Autodesk Inventor part; units mm, degrees
ref_plane "YZ Plane" through (0, 0, 0) normal (1, 0, 0) x (0, 1, 0)
ref_plane "XZ Plane" through (0, 0, 0) normal (0, 1, 0) x (-1, 0, 0)
ref_plane "XY Plane" through (0, 0, 0) normal (0, 0, 1) x (1, 0, 0)
sketch "Sketch1" plane through (0, 0, 0) normal (0, 0, 1) x (1, 0, 0)
  line L0 (-26.9068, 18.7438) -> (-8.9068, 18.7438)
  line L1 (-8.9068, 18.7438) -> (-8.9068, 0.7438)
  line L2 (-8.9068, 0.7438) -> (-26.9068, 0.7438)
  line L3 (-26.9068, 0.7438) -> (-26.9068, 18.7438)
  point P0 (0, 0)
  dimension "d5" = 18
  dimension "d6" = 18
extrude "Extrusion1" add sketch "Sketch1" along normal blind 9
sketch "Sketch2" plane through (0, 0, 0) normal (0, 0, -1) x (-1, 0, 0)
  line L0 (8.9068, 18.7438) -> (26.9068, 18.7438)
  arc A0 (26.9068, 10.7438) -> (18.9068, 18.7438) centre (18.9068, 10.7438) ccw
  arc A1 (25.9068, 10.7438) -> (18.9068, 17.7438) centre (18.9068, 10.7438) ccw
  line L1 (9.9068, 17.7438) -> (25.9068, 17.7438)
  arc A2 (16.9068, 17.7438) -> (9.9068, 10.7438) centre (16.9068, 10.7438) ccw
  arc A3 (16.9068, 18.7438) -> (8.9068, 10.7438) centre (16.9068, 10.7438) ccw
  line L2 (8.9068, 0.7438) -> (8.9068, 18.7438)
  line L3 (9.9068, 1.7438) -> (9.9068, 17.7438)
  arc A4 (8.9068, 8.7438) -> (16.9068, 0.7438) centre (16.9068, 8.7438) ccw
  arc A5 (9.9068, 8.7438) -> (16.9068, 1.7438) centre (16.9068, 8.7438) ccw
  line L4 (26.9068, 0.7438) -> (8.9068, 0.7438)
  line L5 (25.9068, 1.7438) -> (9.9068, 1.7438)
  arc A6 (18.9068, 0.7438) -> (26.9068, 8.7438) centre (18.9068, 8.7438) ccw
  arc A7 (18.9068, 1.7438) -> (25.9068, 8.7438) centre (18.9068, 8.7438) ccw
  line L6 (25.9068, 17.7438) -> (25.9068, 1.7438)
  line L7 (26.9068, 18.7438) -> (26.9068, 0.7438)
  line L8 (26.6568, 10.4938) -> (26.1568, 10.4938)
  line L9 (26.1568, 10.4938) -> (26.1568, 8.9938)
  line L10 (26.1568, 8.9938) -> (26.6568, 8.9938)
  line L11 (26.6568, 8.9938) -> (26.6568, 10.4938)
  circle A8 centre (17.9068, 9.7438) radius 8.75
  line L12 (17.1568, 17.9938) -> (18.6568, 17.9938)
  line L13 (18.6568, 17.9938) -> (18.6568, 18.4938)
  line L14 (18.6568, 18.4938) -> (17.1568, 18.4938)
  line L15 (17.1568, 18.4938) -> (17.1568, 17.9938)
  line L16 (9.6568, 8.9938) -> (9.6568, 10.4938)
  line L17 (9.6568, 10.4938) -> (9.1568, 10.4938)
  line L18 (9.1568, 10.4938) -> (9.1568, 8.9938)
  line L19 (9.1568, 8.9938) -> (9.6568, 8.9938)
  line L20 (18.6568, 1.4938) -> (17.1568, 1.4938)
  line L21 (17.1568, 1.4938) -> (17.1568, 0.9938)
  line L22 (17.1568, 0.9938) -> (18.6568, 0.9938)
  line L23 (18.6568, 0.9938) -> (18.6568, 1.4938)
  point P0 (0, 0)
  point P1 (18.6568, 18.4616)
  point P2 (17.1568, 18.4616)
  point P3 (9.189, 10.4938)
  point P4 (9.189, 8.9938)
  point P5 (17.1568, 1.026)
  point P6 (18.6568, 1.026)
  point P7 (26.6245, 8.9938)
  point P8 (26.6245, 10.4938)
  dimension "d12" = 1.5
  dimension "d13" = 0.5
  dimension "d14" = 0.25
  dimension "d16" = 0.25
  dimension "d18" = 8
  dimension "d19" = 17.5
  dimension "d22" = 360
fillet "Fillet3" radius 8 8 edges at (-8.9068, 18.7438, 4.5) (-17.9068, 18.7438, 9) (-26.9068, 18.7438, 4.5) (-26.9068, 9.7438, 9) (-8.9068, 9.7438, 9) (-8.9068, 0.7438, 4.5) (-17.9068, 0.7438, 9) (-26.9068, 0.7438, 4.5)
shell "Shell2" thickness 1 removed faces 1 at (-17.5734, 12.7438, 0)
extrude "Extrusion4" cut sketch "Sketch2" against normal blind 2 contours A8 L13 L12 L15 | L17 L16 L19 A8 | A8 L10 L9 L8 | L21 L20 L23 A8
properties part number "McCrea_horny_kos_walle_MIR2" material "Silver"
Can you work these out from the model? Positions are in its coordinate system, mm. A direction names the side the tool comes from. Coordinates: 2 decimals unless noted, no trailing zeros. Write each loop counter-clockwise with the first axis right and the second up, starting at its lowest first coordinate (ties: lowest second). Pieces come first, ordered by that corner, then holes. Notation, with made-up numbers: (-28, -38.5) -> (26, -38.5) arc R10 ccw to (26, -19.5) -> close; hole circle Ø5 at (69, -10). An arc over 180 degrees is marked (long way). Answer as CSV lines item,"result".
1) Will these pins go through, and if not, where does the flat tip stop? P1, Ø2, axis at x = -18.5, z = 6, coming from the -Y side; P2, Ø1.6, axis at x = -18, y = 9.5, coming from the -Z side; P3, Ø1.5, axis at x = -19.5, z = 6.5, coming from the +Y side.
Check result:
P1,"y = 1.82"
P2,"z = 8"
P3,"y = 17.16"
2) On a 3-axis mill with a long thin cutter (end or side, diameter ignored), from which of +Z, -Z, +X, -X, +Y, -Y can I reach the whole of each face in a straight line? I mean faces 5 (the cylindrical face through (-17.893, 15.748, 5.895)), 6 (the cylindrical face through (-11.31, 3.03, 0.51)). Say none if no direction works.
Check result:
face 5,"-Z"
face 6,"+Z, -Z, +X, -Y"
3) If we section it at C-C on x = -11.25: Please give me the cut outline in (y, z), then the cut area to 3 significant figures.
Check result:
outline,"(3.09, 0) -> (4.62, 0) -> (4.62, 1) arc R4.12 cw to (8.74, 5.12) -> (10.74, 5.12) arc R4.12 cw to (14.87, 1) -> (14.87, 0) -> (16.4, 0) -> (16.4, 1) arc R5.66 ccw to (10.74, 6.66) -> (8.74, 6.66) arc R5.66 ccw to (3.09, 1) -> close"
area,"29.7 mm²"
4) If we section it at D-D on z = 8.5: Please give me the cut outline in (x, y), then the cut area to 3 significant figures.
Check result:
outline,"(-21.69, 8.74) arc R2.78 ccw to (-18.91, 5.96) -> (-16.91, 5.96) arc R2.78 ccw to (-14.12, 8.74) -> (-14.12, 10.74) arc R2.78 ccw to (-16.91, 13.53) -> (-18.91, 13.53) arc R2.78 ccw to (-21.69, 10.74) -> close"
area,"50.6 mm²"
5) If I drill on line 1 (X direction, y = 10.75, z = 6.25); line 2 (X direction, y = 14.25, z = 5.5); line 3 (Y direction, x = -17.75, z = 3.5), over which ranges is the centre line in solid material (lowest first)? Write a range as from..to.
Check result:
line 1,"-24.94..-23.54, -12.28..-10.87"
line 2,"-24.52..-22.96, -12.85..-11.3"
line 3,"1.14..2.21, 17.28..18.34"
6) If we mould it in two halves opening along X, with no side actions, what happens to faces 1 (the flat face through (-26.157, 10, 1)), 2 (the cylindrical face through (-11.19, 16.34, 0.51)), 3 (the cylindrical face through (-17.921, 3.74, 5.895)), 4 (the flat face through (-19, 18, 0))? For each: +X half, -X half, draft (parallel to the pull), parting line (faces both ways), or undercut.
Check result:
face 1,"undercut"
face 2,"+X half"
face 3,"undercut"
face 4,"draft"
7) If we section it at B-B on z = 2.25: Please give me the cut outline in (x, y).
Check result:
outline,"(-26.81, 8.74) arc R7.9 ccw to (-18.91, 0.84) -> (-16.91, 0.84) arc R7.9 ccw to (-9.01, 8.74) -> (-9.01, 10.74) arc R7.9 ccw to (-16.91, 18.65) -> (-18.91, 18.65) arc R7.9 ccw to (-26.81, 10.74) -> close; hole (-25.79, 8.74) arc R6.89 ccw to (-18.91, 1.86) -> (-16.91, 1.86) arc R6.89 ccw to (-10.02, 8.74) -> (-10.02, 10.74) arc R6.89 ccw to (-16.91, 17.63) -> (-18.91, 17.63) arc R6.89 ccw to (-25.79, 10.74) -> close"
8) If we section it at A-A on y = 15.5: Please give me the cut outline in (x, z).
Check result:
outline,"(-25.34, 0) -> (-24.04, 0) -> (-24.04, 1) arc R5.14 cw to (-18.91, 6.14) -> (-16.91, 6.14) arc R5.14 cw to (-11.77, 1) -> (-11.77, 0) -> (-10.47, 0) -> (-10.47, 1) arc R6.43 ccw to (-16.91, 7.43) -> (-18.91, 7.43) arc R6.43 ccw to (-25.34, 1) -> close"
